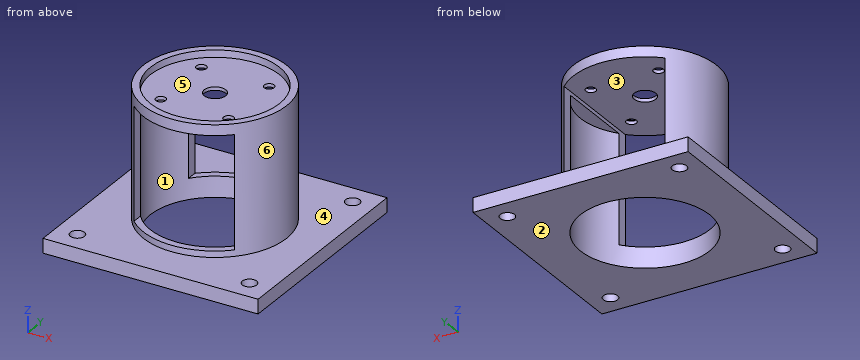
Autodesk Fusion 360 part; units mm, degrees
sketch "Sketch1" plane through (0, 0, 0) normal (0, 0, 1) x (1, 0, 0)
  line L0 (75, 75) -> (-75, 75)
  line L1 (-75, 75) -> (-75, -75)
  line L2 (-75, -75) -> (75, -75)
  line L3 (75, -75) -> (75, 75)
  line L4 (75, 75) -> (-75, -75) construction
  line L5 (-75, 75) -> (75, -75) construction
  circle A0 centre (-60, 60) radius 5
  circle A1 centre (60, 60) radius 5
  circle A2 centre (-60, -60) radius 5
  circle A3 centre (60, -60) radius 5
  circle A4 centre (0, 0) radius 50
  circle A5 centre (0, 0) radius 45
  dimension "d1" = 150
  dimension "d2" = 150
  dimension "d3" = 10
  dimension "d4" = 10
  dimension "d5" = 10
  dimension "d6" = 10
  dimension "d7" = 100
  dimension "d8" = 90
extrude "Extrude1" add sketch "Sketch1" along normal blind 10 contours L0 L1 L2 L3
extrude "Extrude2" add sketch "Sketch1" along normal blind 100 contours A4
extrude "Extrude3" add sketch "Sketch1" along normal blind 95 contours A5
extrude "Extrude4" cut sketch "Sketch1" along normal blind 90 contours A5
sketch "Sketch2" plane through (0, 0, 95) normal (0, 0, 1) x (-1, 0, 0)
  circle A0 centre (0, 0) radius 45
  circle A1 centre (0, 0) radius 7.5
  dimension "d17" = 15
extrude "Extrude5" cut sketch "Sketch2" against normal blind 10 contours A1
sketch "Sketch3" plane through (0, 0, 0) normal (0, 1, 0) x (1, 0, 0)
  line L0 (35.1024, -92.6698) -> (-35.2945, -92.6698)
  line L1 (-35.2945, -92.6698) -> (-35.2945, -14.3779)
  line L2 (-35.2945, -14.3779) -> (35.1024, -14.3779)
  line L3 (35.1024, -14.3779) -> (35.1024, -92.6698)
  line L4 (35.1024, -92.6698) -> (-35.2945, -14.3779) construction
  line L5 (-35.2945, -92.6698) -> (35.1024, -14.3779) construction
  point P0 (-0.096, -53.5238)
extrude "Extrude6" cut sketch "Sketch3" along normal mid plane 120
sketch "Sketch4" plane through (0, 0, 95) normal (0, 0, 1) x (-1, 0, 0)
  line L0 (23.622, 23.622) -> (-23.622, 23.622)
  line L1 (-23.622, 23.622) -> (-23.622, -23.622)
  line L2 (-23.622, -23.622) -> (23.622, -23.622)
  line L3 (23.622, -23.622) -> (23.622, 23.622)
  line L4 (23.622, 23.622) -> (-23.622, -23.622) construction
  line L5 (-23.622, 23.622) -> (23.622, -23.622) construction
  circle A0 centre (23.622, 23.622) radius 3.5
  circle A1 centre (-23.622, 23.622) radius 3.5
  circle A2 centre (23.622, -23.622) radius 3.5
  circle A3 centre (-23.622, -23.622) radius 3.5
  dimension "d22" = 47.244
  dimension "d23" = 47.244
  dimension "d24" = 7
  dimension "d25" = 7
  dimension "d26" = 7
  dimension "d27" = 7
extrude "Extrude7" cut sketch "Sketch4" against normal blind 10 contours L0 L1 A1 | L0 L1 A1 | L0 L3 A0 | L0 L3 A0 | L1 L2 A3 | L1 L2 A3 | L2 L3 A2 | L2 L3 A2
Geometry: final body of the model. Coordinates: model frame, mm. Face numbers are marked on the shaded views. A direction names the side the tool comes from. Round coordinates to 2 decimals unless told otherwise and drop trailing zeros. Loops run counter-clockwise (first coordinate to the right, second up) from the corner with the lowest first, then second, coordinate; pieces in that order, holes last. Notation, with made-up numbers: (81.5, 67.25) - (85.5, 67.25) arc R16 ccw to (85.5, 86.25) - close; hole circle Ø11 at (13.25, 59). An arc over 180 degrees is marked (long way). Write each question's results on one line, items separated by ' | '. Start each with the question number.
1) First-contact query: P1, Ø8, axis at x = 12, y = -54.5, coming from the +Z side; P2, Ø10, axis at x = -13, y = -2, coming from the +Z side; P3, Ø5, axis at x = 39, y = 10, coming from the -Z side. Flat tips, straight axial feed; report the tip coordinate or a pass-through.
2) Mould query, pull axis Y, two halves, no side actions, for the marked faces 4, 5 and 6. Classes: released by +Y, released by -Y, zero draft, split by the parting line, or undercut.
3) Cut plane B-B on x = 57. Return loops of the section in (y, z), then the cut area to 3 significant figures.
4) Cut plane C-C on z = 64. Return loops of the section in (x, y).
5) Cut plane A-A on y = 0. Return loops of the section in (x, z).
6) Cut plane D-D on y = 60. Return loops of the section in (x, z), then the cut area to 3 significant figures.
7) Access query for the marked faces 1, 2 and 3. Directions: +Z, -Z, +X, -X, +Y, -Y. A direction counts if a zero-diameter tool reaches every point of the face in a straight line with its end or side. Return the directions, or none.
8) Line query: probe 1 along Y at (x, z) = (60, 3); probe 2 along Z at (x, y) = (-14.5, 43); probe 3 along Y at (x, z) = (-39, 95.5). Output: solid intervals per line, ascending. Write a range as [from, to].
Verdict:
1) P1: stops at z = 10 | P2: stops at z = 95 | P3: stops at z = 90
2) face 4: zero draft | face 5: undercut | face 6: split by the parting line
3) outline: (-75, 0) - (-64, 0) - (-64, 10) - (-75, 10) - close; (-56, 0) - (56, 0) - (56, 10) - (-56, 10) - close; (64, 0) - (75, 0) - (75, 10) - (64, 10) - close | area: 1,340 mm2
4) outline: (-35.29, -35.42) - (-35.29, -27.92) arc R45 cw to (-35.29, 27.92) - (-35.29, 35.42) arc R50 ccw to start; (35.1, -35.61) arc R50 ccw to (35.1, 35.61) - (35.1, 28.16) arc R45 cw to (35.1, -28.16) - close
5) outline: (-75, 0) - (-45, 0) - (-45, 90) - (-35.29, 90) - (-35.29, 92.67) - (-7.5, 92.67) - (-7.5, 95) - (-45, 95) - (-45, 100) - (-50, 100) - (-50, 10) - (-75, 10) - close; (7.5, 92.67) - (35.1, 92.67) - (35.1, 90) - (45, 90) - (45, 0) - (75, 0) - (75, 10) - (50, 10) - (50, 100) - (45, 100) - (45, 95) - (7.5, 95) - close
6) outline: (-75, 0) - (-65, 0) - (-65, 10) - (-75, 10) - close; (-55, 0) - (55, 0) - (55, 10) - (-55, 10) - close; (65, 0) - (75, 0) - (75, 10) - (65, 10) - close | area: 1,300 mm2
7) face 1: -Z | face 2: -Z, +X, -X, +Y, -Y | face 3: +Y, -Y
8) probe 1: y = [-75, -65], [-55, 55], [65, 75] | probe 2: z = [0, 14.38], [92.67, 100] | probe 3: y = [-31.29, -22.45], [22.45, 31.29]
